For this review, take the finished solid that the model builds, in its own axes (mm). Face numbers are marked on the shaded views. A direction names the side the tool comes from. Coordinates: 2 decimals unless noted, no trailing zeros.
1. To check wall thickness, follow probe 1 along X at (y, z) = (15, 3.25); probe 2 along Y at (x, z) = (-14, 1); probe 3 along Y at (x, z) = (16, 4). State the ranges of each line that lie inside material, in increasing order.
2. Machinability: for the marked faces 4, 5, 6 and 7, which of the approach directions +Z, -Z, +X, -X, +Y, -Y give a long, thin tool a straight path to every point of the face, cutting with its end or side? Answer none if there is none.
3. Mouldability with a two-part tool opening along X and no side actions: class the marked faces 1, 2 and 3 as pulls with the +X half, pulls with the -X half, needs draft (parallel to the pull), parting line crosses it, or undercut.
4. Clearance check with flat-ended pins moving along their axes: P1, Ø8, axis at x = -1, y = 4, coming from the -Z side; P2, Ø4, axis at y = -1.5, z = 6.5, coming from the -X side; P3, Ø5, axis at x = 4, z = 4.5, coming from the +Y side; P4, Ø1.5, axis at y = 7, z = 5, coming from the +X side. State where each tip first meets the part, or that it passes through.
```python
from build123d import *

# Parameters (mm, degrees)
F1_DEPTH = 10


with BuildPart() as f1:
    # F0 (on Top) → F1 (new body)
    with BuildSketch(Plane.XY):
        with BuildLine():
            ThreePointArc((0.834247, 13.754724), (0.539473, 13.922611), (0.384061, 14.224148))
            ThreePointArc((0.384061, 14.224148), (-0.053041, 16.126356), (-1.146638, 17.742988))
            Line((-1.146638, 17.742988), (-1.950006, 17.672744))
            ThreePointArc((-1.950006, 17.672744), (-2.74627, 15.891587), (-2.846993, 13.943148))
            ThreePointArc((-2.846993, 13.943148), (-2.94723, 13.618388), (-3.20868, 13.401223))
            Line((-3.20868, 13.401223), (-3.920457, 13.210542))
            ThreePointArc((-3.920457, 13.210542), (-4.254874, 13.267486), (-4.504046, 13.497684))
            ThreePointArc((-4.504046, 13.497684), (-5.565381, 15.135677), (-7.145946, 16.280782))
            Line((-7.145946, 16.280782), (-7.876841, 15.940006))
            ThreePointArc((-7.876841, 15.940006), (-8.015892, 13.993927), (-7.444136, 12.128545))
            ThreePointArc((-7.444136, 12.128545), (-7.427254, 11.789086), (-7.598661, 11.495597))
            Line((-7.598661, 11.495597), (-8.202296, 11.072974))
            ThreePointArc((-8.202296, 11.072974), (-8.536021, 11.012106), (-8.848898, 11.1432))
            ThreePointArc((-8.848898, 11.1432), (-10.406453, 12.319412), (-12.283348, 12.854873))
            Line((-12.283348, 12.854873), (-12.853612, 12.284668))
            ThreePointArc((-12.853612, 12.284668), (-12.31868, 10.408393), (-11.143406, 8.85106))
            ThreePointArc((-11.143406, 8.85106), (-11.01144, 8.537847), (-11.072132, 8.203432))
            Line((-11.072132, 8.203432), (-11.494817, 7.599841))
            ThreePointArc((-11.494817, 7.599841), (-11.787598, 7.428503), (-12.126443, 7.444681))
            ThreePointArc((-12.126443, 7.444681), (-13.992354, 8.017243), (-15.939197, 7.878477))
            Line((-15.939197, 7.878477), (-16.280048, 7.147617))
            ThreePointArc((-16.280048, 7.147617), (-15.135653, 5.567454), (-13.498617, 4.506006))
            ThreePointArc((-13.498617, 4.506006), (-13.267485, 4.256818), (-13.21014, 3.921813))
            Line((-13.21014, 3.921813), (-13.400893, 3.210056))
            ThreePointArc((-13.400893, 3.210056), (-13.617417, 2.948914), (-13.94136, 2.848224))
            ThreePointArc((-13.94136, 2.848224), (-15.890571, 2.748077), (-17.672544, 1.95182))
            Line((-17.672544, 1.95182), (-17.74287, 1.148459))
            ThreePointArc((-17.74287, 1.148459), (-16.127043, 0.054997), (-14.225696, -0.382538))
            ThreePointArc((-14.225696, -0.382538), (-13.923275, -0.537647), (-13.75481, -0.832836))
            Line((-13.75481, -0.832836), (-13.690624, -1.566909))
            ThreePointArc((-13.690624, -1.566909), (-13.804774, -1.886358), (-14.074743, -2.091771))
            ThreePointArc((-14.074743, -2.091771), (-15.87215, -2.852547), (-17.274321, -4.210255))
            Line((-17.274321, -4.210255), (-17.06564, -4.989221))
            ThreePointArc((-17.06564, -4.989221), (-15.173273, -5.464093), (-13.236946, -5.224943))
            ThreePointArc((-13.236946, -5.224943), (-12.899713, -5.267264), (-12.640446, -5.487031))
            Line((-12.640446, -5.487031), (-12.329064, -6.154883))
            ThreePointArc((-12.329064, -6.154883), (-12.327072, -6.494108), (-12.510505, -6.779467))
            ThreePointArc((-12.510505, -6.779467), (-13.939314, -8.109113), (-14.79256, -9.864511))
            Line((-14.79256, -9.864511), (-14.330042, -10.525127))
            ThreePointArc((-14.330042, -10.525127), (-12.389383, -10.324133), (-10.651624, -9.437142))
            ThreePointArc((-10.651624, -9.437142), (-10.320255, -9.36157), (-10.001459, -9.47941))
            Line((-10.001459, -9.47941), (-9.480437, -10.000486))
            ThreePointArc((-9.480437, -10.000486), (-9.362542, -10.318572), (-9.437314, -10.64946))
            ThreePointArc((-9.437314, -10.64946), (-10.32519, -12.387599), (-10.526598, -14.328962))
            Line((-10.526598, -14.328962), (-9.86603, -14.791547))
            ThreePointArc((-9.86603, -14.791547), (-8.11115, -13.93893), (-6.78156, -12.511083))
            ThreePointArc((-6.78156, -12.511083), (-6.496022, -12.326734), (-6.156148, -12.328432))
            Line((-6.156148, -12.328432), (-5.488329, -12.639883))
            ThreePointArc((-5.488329, -12.639883), (-5.268753, -12.898464), (-5.225845, -13.234971))
            ThreePointArc((-5.225845, -13.234971), (-5.465697, -15.171959), (-4.990972, -17.065128))
            Line((-4.990972, -17.065128), (-4.212028, -17.273888))
            ThreePointArc((-4.212028, -17.273888), (-2.854593, -15.872486), (-2.093539, -14.076003))
            ThreePointArc((-2.093539, -14.076003), (-1.888272, -13.805111), (-1.568315, -13.690463))
            Line((-1.568315, -13.690463), (-0.834247, -13.754724))
            ThreePointArc((-0.834247, -13.754724), (-0.539473, -13.922611), (-0.384061, -14.224148))
            ThreePointArc((-0.384061, -14.224148), (0.053041, -16.126356), (1.146638, -17.742988))
            Line((1.146638, -17.742988), (1.950006, -17.672744))
            ThreePointArc((1.950006, -17.672744), (2.74627, -15.891587), (2.846993, -13.943148))
            ThreePointArc((2.846993, -13.943148), (2.94723, -13.618388), (3.20868, -13.401223))
            Line((3.20868, -13.401223), (3.920457, -13.210542))
            ThreePointArc((3.920457, -13.210542), (4.254874, -13.267486), (4.504046, -13.497684))
            ThreePointArc((4.504046, -13.497684), (5.565381, -15.135677), (7.145946, -16.280782))
            Line((7.145946, -16.280782), (7.876841, -15.940006))
            ThreePointArc((7.876841, -15.940006), (8.015892, -13.993927), (7.444136, -12.128545))
            ThreePointArc((7.444136, -12.128545), (7.427254, -11.789086), (7.598661, -11.495597))
            Line((7.598661, -11.495597), (8.202296, -11.072974))
            ThreePointArc((8.202296, -11.072974), (8.536021, -11.012106), (8.848898, -11.1432))
            ThreePointArc((8.848898, -11.1432), (10.406453, -12.319412), (12.283348, -12.854873))
            Line((12.283348, -12.854873), (12.853612, -12.284668))
            ThreePointArc((12.853612, -12.284668), (12.31868, -10.408393), (11.143406, -8.85106))
            ThreePointArc((11.143406, -8.85106), (11.01144, -8.537847), (11.072132, -8.203432))
            Line((11.072132, -8.203432), (11.494817, -7.599841))
            ThreePointArc((11.494817, -7.599841), (11.787598, -7.428503), (12.126443, -7.444681))
            ThreePointArc((12.126443, -7.444681), (13.992354, -8.017243), (15.939197, -7.878477))
            Line((15.939197, -7.878477), (16.280048, -7.147617))
            ThreePointArc((16.280048, -7.147617), (15.135653, -5.567454), (13.498617, -4.506006))
            ThreePointArc((13.498617, -4.506006), (13.267485, -4.256818), (13.21014, -3.921813))
            Line((13.21014, -3.921813), (13.400893, -3.210056))
            ThreePointArc((13.400893, -3.210056), (13.617417, -2.948914), (13.94136, -2.848224))
            ThreePointArc((13.94136, -2.848224), (15.890571, -2.748077), (17.672544, -1.95182))
            Line((17.672544, -1.95182), (17.74287, -1.148459))
            ThreePointArc((17.74287, -1.148459), (16.127043, -0.054997), (14.225696, 0.382538))
            ThreePointArc((14.225696, 0.382538), (13.923275, 0.537647), (13.75481, 0.832836))
            Line((13.75481, 0.832836), (13.690624, 1.566909))
            ThreePointArc((13.690624, 1.566909), (13.804774, 1.886358), (14.074743, 2.091771))
            ThreePointArc((14.074743, 2.091771), (15.87215, 2.852547), (17.274321, 4.210255))
            Line((17.274321, 4.210255), (17.06564, 4.989221))
            ThreePointArc((17.06564, 4.989221), (15.173273, 5.464093), (13.236946, 5.224943))
            ThreePointArc((13.236946, 5.224943), (12.899713, 5.267264), (12.640446, 5.487031))
            Line((12.640446, 5.487031), (12.329064, 6.154883))
            ThreePointArc((12.329064, 6.154883), (12.327072, 6.494108), (12.510505, 6.779467))
            ThreePointArc((12.510505, 6.779467), (13.939314, 8.109113), (14.79256, 9.864511))
            Line((14.79256, 9.864511), (14.330042, 10.525127))
            ThreePointArc((14.330042, 10.525127), (12.389383, 10.324133), (10.651624, 9.437142))
            ThreePointArc((10.651624, 9.437142), (10.320255, 9.36157), (10.001459, 9.47941))
            Line((10.001459, 9.47941), (9.480437, 10.000486))
            ThreePointArc((9.480437, 10.000486), (9.362542, 10.318572), (9.437314, 10.64946))
            ThreePointArc((9.437314, 10.64946), (10.32519, 12.387599), (10.526598, 14.328962))
            Line((10.526598, 14.328962), (9.86603, 14.791547))
            ThreePointArc((9.86603, 14.791547), (8.11115, 13.93893), (6.78156, 12.511083))
            ThreePointArc((6.78156, 12.511083), (6.496022, 12.326734), (6.156148, 12.328432))
            Line((6.156148, 12.328432), (5.488329, 12.639883))
            ThreePointArc((5.488329, 12.639883), (5.268753, 12.898464), (5.225845, 13.234971))
            ThreePointArc((5.225845, 13.234971), (5.465697, 15.171959), (4.990972, 17.065128))
            Line((4.990972, 17.065128), (4.212028, 17.273888))
            ThreePointArc((4.212028, 17.273888), (2.854593, 15.872486), (2.093539, 14.076003))
            ThreePointArc((2.093539, 14.076003), (1.888272, 13.805111), (1.568315, 13.690463))
            Line((1.568315, 13.690463), (0.834247, 13.754724))
        make_face()
        Polygon((8.873521, 3.204124), (8.037635, -4.93986), (1.149246, -9.364028), (-6.604549, -6.736893), (-9.384984, 0.96326), (-5.098334, 7.938059), (3.027465, 8.935337), align=None, mode=Mode.SUBTRACT)
    extrude(amount=F1_DEPTH)


solid = f1.part
```
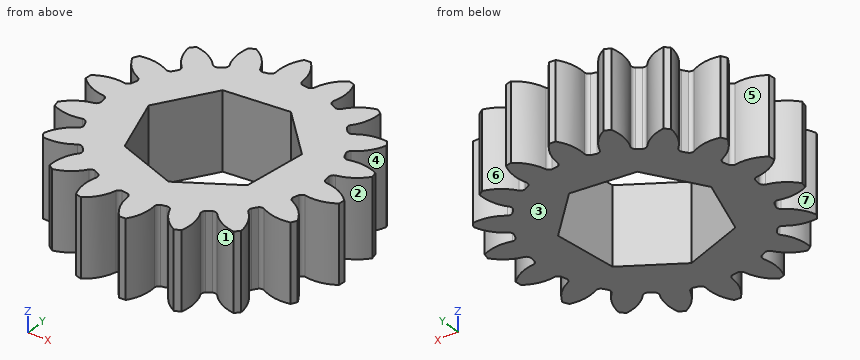
Results list:
1. probe 1: x = -8.03 to -5.44, -2.88 to 0.29, 2.39 to 5.47
1. probe 2: y = -10.54 to -8.19, -5.41 to -2.06, -0.48 to 2.86, 4.74 to 8.02
1. probe 3: y = -7.75 to -6.63, -2.72 to 0, 2.94 to 5.35
2. face 4: +Z, -Z, +X
2. face 5: +Z, -Z
2. face 6: +Z, -Z, +Y
2. face 7: +Z, -Z, -X
3. face 1: undercut
3. face 2: pulls with the +X half
3. face 3: needs draft
4. P1: passes through
4. P2: stops at x = -16.95
4. P3: stops at y = 17.27
4. P4: stops at x = 13.65
